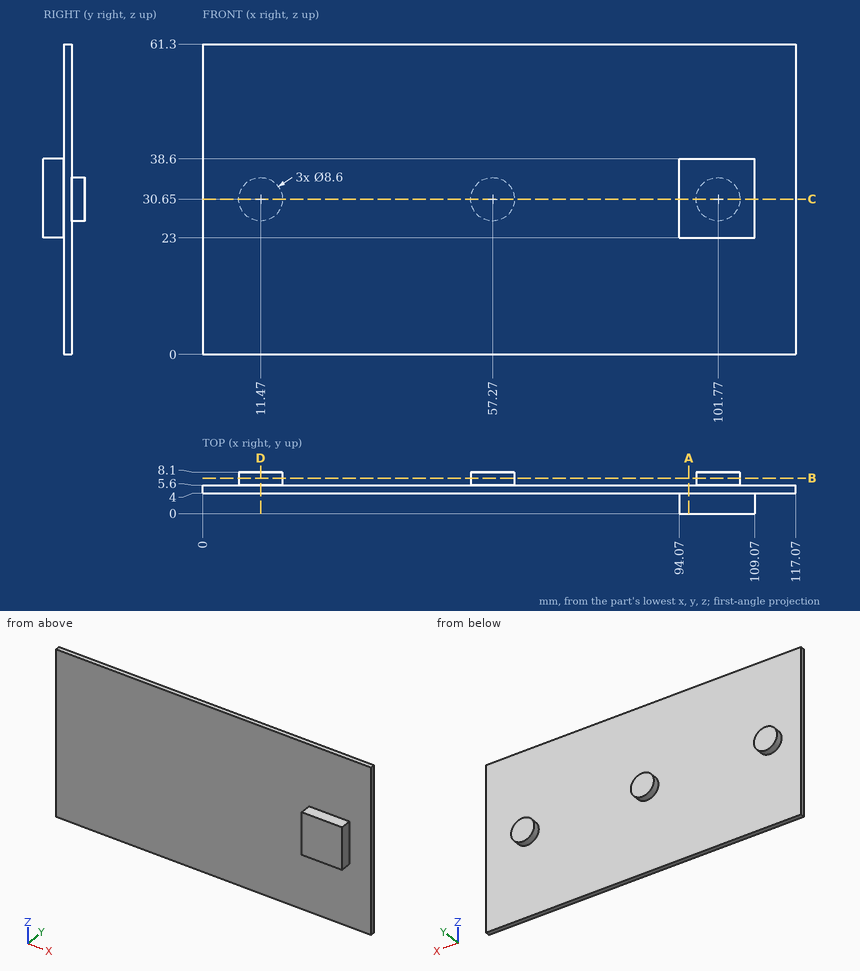
Study the drawing (mm; zero at the part's minimum x, y, z) and answer. Give positions to 0.01 mm unless a question says otherwise; leave off trailing zeros. Order: outer loops, then holes, each group sorted by start corner. A loop starts at its lowest first (then second) coordinate and runs counter-clockwise, first axis right, second up. Notation, with made-up numbers: (12, 89.5) - (53, 89.5) arc R9 cw to (53, 96.5) - close; hole circle Ø6 at (42.5, -37.75). An arc over 180 degrees is marked (long way). Use one line per item in the form item = value. Start each with the question number.
(1) A cutting plane is placed at C-C, the plane z = 30.65. Write down the section's boundary in (x, y), then the cut area to 3 significant figures.
(2) Flat-ended cylindrical pins translate along their axes: pin 1 Ø18.5 at (x, z) = (43, 33) entering from -Y; pin 2 Ø4.5 at (x, y) = (104, 1) entering from -Z; pin 3 Ø4.5 at (y, z) = (1.5, 34) entering from +X. Find the tip coordinate at first contact, or state that the pin passes through.
(3) A cutting plane is placed at A-A, the plane x = 96. Write down the section's boundary in (y, z), then the cut area to 3 significant figures.
(4) A cutting plane is placed at B-B, the plane y = 7. Write down the section's boundary in (x, z), then the cut area to 3 significant figures.
(5) A cutting plane is placed at D-D, the plane x = 11.47. Write down the section's boundary in (y, z).
(6) Consider line 1 (Z direction, x = 103, y = 1.75); line 2 (Y direction, x = 90, z = 35.5); line 3 (X direction, y = 7.75, z = 29.5). Determine where each line is inside the solid, lowest interval first. Write a range as from..to.
Ans:
q1.outline = (0, 4) - (94.07, 4) - (94.07, 0) - (109.07, 0) - (109.07, 4) - (117.07, 4) - (117.07, 5.6) - (106.07, 5.6) - (106.07, 8.1) - (97.47, 8.1) - (97.47, 5.6) - (61.57, 5.6) - (61.57, 8.1) - (52.97, 8.1) - (52.97, 5.6) - (15.77, 5.6) - (15.77, 8.1) - (7.17, 8.1) - (7.17, 5.6) - (0, 5.6) - close
q1.area = 312 mm^2
q2.pin_1 = 4
q2.pin_2 = 23
q2.pin_3 = 109.07
q3.outline = (0, 23) - (4, 23) - (4, 0) - (5.6, 0) - (5.6, 61.3) - (4, 61.3) - (4, 38.6) - (0, 38.6) - close
q3.area = 160 mm^2
q4.outline = circle Ø8.6 at (11.47, 30.65); circle Ø8.6 at (57.27, 30.65); circle Ø8.6 at (101.77, 30.65)
q4.area = 174 mm^2
q5.outline = (4, 0) - (5.6, 0) - (5.6, 26.35) - (8.1, 26.35) - (8.1, 34.95) - (5.6, 34.95) - (5.6, 61.3) - (4, 61.3) - close
q6.line_1 = 23..38.6
q6.line_2 = 4..5.6
q6.line_3 = 7.33..15.61, 53.13..61.41, 97.63..105.91
